Answer from the drawing. Dimensions are ordinates in mm from the lowest x, y and z of the part. A direction names the side the tool comes from. Round coordinates to 2 decimals unless told otherwise and drop trailing zeros. Write each loop counter-clockwise with the first axis right and the second up, starting at its lowest first coordinate (ties: lowest second). Pieces come first, ordered by that corner, then holes.
1. Find section A-A (z = 11). Write down the section's boundary in (x, y).
2. Find section C-C (x = 7.8). Write down the section's boundary in (y, z).
3. Find section B-B (y = 1.2). Write down the section's boundary in (x, z), and give its area (3 significant figures).
4. Find section D-D (x = 5). Write down the section's boundary in (y, z), and give its area (3 significant figures).
5. A tool of negligible diameter and unlimited length cuts with its end or side. For the marked faces 4, 5 and 6, from which of +Z, -Z, +X, -X, +Y, -Y can it reach the whole face along a straight path? Write none if from no direction.
6. Straight lines are drawn through the part: probe 1 along X at (y, z) = (0.7, 5); probe 2 along Y at (x, z) = (5, 11.5); probe 3 along X at (y, z) = (4.7, 9). For each, find the intervals that lie inside material, in ascending order.
7. Flat-ended cylindrical pins translate along their axes: pin 1 Ø1.6 at (y, z) = (1, 6) entering from +X; pin 2 Ø1.5 at (x, z) = (4.5, 4) entering from +Y; pin 3 Ø0.6 at (x, z) = (4.5, 4.5) entering from -Y. Find the tip coordinate at first contact, or state that the pin passes through.
8. Determine the mould class of the marked faces 1, 2 and 3 for opening direction X: pulls with the +X half, pulls with the -X half, needs draft (parallel to the pull), parting line crosses it, or undercut.
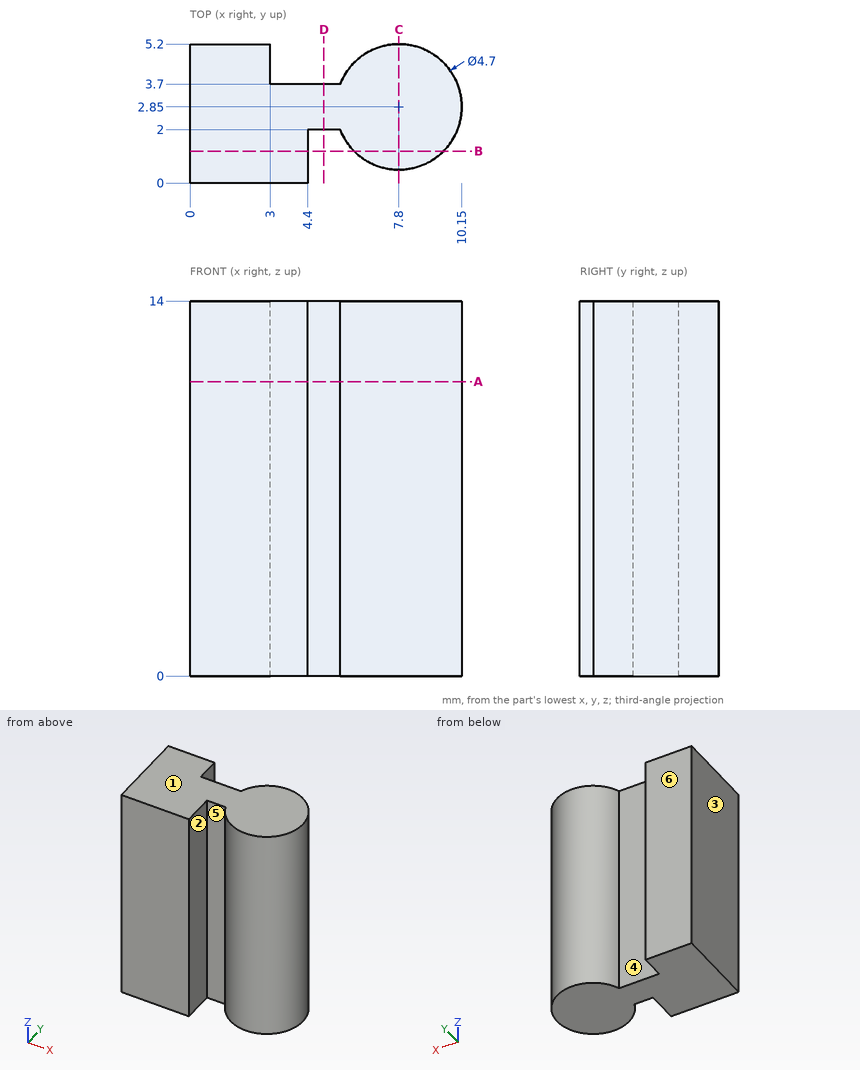
Worked answers:
1. outline: (0, 0) - (4.4, 0) - (4.4, 2) - (5.61, 2) arc R2.35 ccw (long way) to (5.61, 3.7) - (3, 3.7) - (3, 5.2) - (0, 5.2) - close
2. outline: (0.5, 0) - (5.2, 0) - (5.2, 14) - (0.5, 14) - close
3. outline: (0, 0) - (4.4, 0) - (4.4, 14) - (0, 14) - close; (6.13, 0) - (9.47, 0) - (9.47, 14) - (6.13, 14) - close
3. area: 108 mm2
4. outline: (2, 0) - (3.7, 0) - (3.7, 14) - (2, 14) - close
4. area: 23.8 mm2
5. face 4: +Z, -Z, +Y
5. face 5: +Z, -Z, -Y
5. face 6: +Z, -Z, +X, -X, +Y
6. probe 1: x = 0 to 4.4, 6.85 to 8.75
6. probe 2: y = 2 to 3.7
6. probe 3: x = 0 to 3, 6.35 to 9.25
7. pin 1: stops at x = 9.9
7. pin 2: stops at y = 3.7
7. pin 3: stops at y = 0
8. face 1: needs draft
8. face 2: undercut
8. face 3: pulls with the -X half
